from build123d import *

# Parameters (mm, degrees)
F0_R          = 9.525
F1_DEPTH      = 25.4
F1_DEPTH_BACK = 25.4
F3_D          = 12
F3_DEPTH      = 25.401
F4_SIZE       = 1.27
F6_D          = 2.7178
F6_DEPTH      = 9.526


with BuildPart() as f1:
    # F0 (on Front) → F1 (new body, two sides)
    with BuildSketch(Plane.XZ) as f1_sk:
        Circle(F0_R)
    extrude(amount=F1_DEPTH)
    extrude(f1_sk.sketch, amount=-F1_DEPTH_BACK)

    # F3 (through all, one way)
    with BuildSketch(Plane(origin=(0, 0, 0), x_dir=(1, 0, 0), z_dir=(0, 1, 0))):
        with Locations((0, 0)):
            Circle(F3_D / 2)
    extrude(amount=-F3_DEPTH, mode=Mode.SUBTRACT)

    # F4
    f4_edges = [f1.edges().sort_by_distance(p)[0] for p in [
        (-9.525, -25.4, 0),
        (-9.525, 25.4, 0),
    ]]
    chamfer(f4_edges, length=F4_SIZE)

    # F6 (through all, one way)
    with BuildSketch(Plane(origin=(0, 0, 0), x_dir=(1, 0, 0), z_dir=(0, 0, -1))):
        with Locations((0, -20.32), (0, 20.32)):
            Circle(F6_D / 2)
    extrude(amount=-F6_DEPTH, mode=Mode.SUBTRACT)


solid = f1.part
Read the model definition and answer for the solid it produces. Units are mm, in the model's axes. A direction names the side the tool comes from. Round coordinates to 2 decimals unless told otherwise and drop trailing zeros. Loops run counter-clockwise (first coordinate to the right, second up) from the corner with the lowest first, then second, coordinate; pieces in that order, holes last. Notation, with made-up numbers: (60.5, 81) - (95.5, 81) arc R11 ccw to (95.5, 102) - close; hole circle Ø9 at (20, 75.25). An arc over 180 degrees is marked (long way). One line per question, with ' | ' between items. Start each with the question number.
Q1. Section B-B on y = -18.5 is taken. Give the vertices of the cut face in (x, z) (3 decimals), plus the area to 3 significant figures.
Q2. For faces 4 (the flat face through (0, 0, 0)), 5 (the flat face through (-4, -25.4, -5)), 6 (the cylindrical face through (-0.295, 21.647, 4.697)), determine the directions among +Z, -Z, +X, -X, +Y, -Y from which every point of the face is accessible in a straight line to the end or side of a thin tool.
Q3. Section A-A on x = 0 is taken. Give the vertices of the cut face in (y, z) (3 decimals), plus the area to 3 significant figures.
Q4. Flat-ended cylindrical pins translate along their axes: pin 1 (1 mm diameter, centred on y = 15.5, z = -7.5, fed in from +X); pin 2 (10 mm diameter, centred on x = -7.5, y = 8, fed in from -Z); pin 3 (0.8 mm diameter, centred on x = 0, y = 20.5, fed in from +Z). Find the tip coordinate at first contact, or state that the pin passes through.
Q5. Section D-D on y = 20.32 is taken. Give the vertices of the cut face in (x, z) (3 decimals).
Q6. Find the intervals of material crossed by L1, parallel to Y at x = 0, z = 8.1; L2, parallel to Z at x = 0, y = -8.75 (3 decimals); L3, parallel to Y at x = 0, z = 3.75, in increasing order.
Q7. For a pull along Z with two mould halves and no side action, classify faces 1 (the cylindrical face through (-6, -13, 0)), 2 (the cylindrical face through (-7.559, -0.338, -5.796)), 3 (the cylindrical face through (-0.295, -18.993, 7.658)) as +Z half, -Z half, draft (parallel to the pull), parting line (faces both ways), or undercut.
Q8. Section C-C on y = 5.5 is taken. Give the vertices of the cut face in (x, z) (3 decimals), plus the area to 3 significant figures.
Established:
1) outline: circle Ø19.05 at (0, 0); hole circle Ø12 at (0, 0) | area: 172 mm²
2) face 4: -Y | face 5: +Z, -Z, +X, -X, -Y | face 6: +Z
3) outline: (-25.4, -8.255) - (-24.13, -9.525) - (24.13, -9.525) - (25.4, -8.255) - (25.4, 8.255) - (24.13, 9.525) - (21.679, 9.525) - (21.679, 0) - (18.961, 0) - (18.961, 9.525) - (-18.961, 9.525) - (-18.961, 6) - (0, 6) - (0, -6) - (-25.4, -6) - close; (-25.4, 6) - (-21.679, 6) - (-21.679, 9.525) - (-24.13, 9.525) - (-25.4, 8.255) - close | area: 624 mm²
4) pin 1: x = 6.46 | pin 2: z = -9.19 | pin 3: z = 0
5) outline: (-1.359, 0) - (-1.359, 9.428) arc R9.525 ccw (long way) to (1.359, 9.428) - (1.359, 0) - close
6) L1: -25.4 to -21.68, -18.96 to 18.96, 21.68 to 25.4 | L2: -9.525 to -6, 6 to 9.525 | L3: 0 to 18.96, 21.68 to 25.4
7) face 1: undercut | face 2: parting line | face 3: draft
8) outline: circle Ø19.05 at (0, 0) | area: 285 mm²
